The model under review builds one solid part; all positions refer to its coordinate system, in mm. Face numbers are marked on the shaded views. A direction names the side the tool comes from. Coordinates: 2 decimals unless noted, no trailing zeros. Order: outer loops, then holes, each group sorted by start corner. A loop starts at its lowest first (then second) coordinate and runs counter-clockwise, first axis right, second up. Notation, with made-up numbers: M 23.25,-21 L 46.25,-21 A21 cw 46.25,9 Z; hole C -9,78.5 d10. An arc over 180 degrees is marked long. One line per item, written item: value.
```python
from build123d import *

# Parameters (mm, degrees)
BOSS_EXTRUDE1_DEPTH        = 12.5
FILLET1_R                  = 2
F_3_5_3_5_DIAMETER_HOLE1_D = 3.5


with BuildPart() as part:
    # Sketch1 → Boss-Extrude1 (new body, symmetric)
    with BuildSketch(Plane.XY):
        Polygon((0, 0), (-18, 0), (-18, -5.5), (-35, -5.5), (-35, -3.5), (-20, -3.5), (-20, 2), (0, 2), align=None)
    extrude(amount=BOSS_EXTRUDE1_DEPTH, both=True)

    # Fillet1
    fillet1_edges = [part.edges().sort_by_distance(p)[0] for p in [
        (-18, -5.5, 0),
        (-20, 2, 0),
    ]]
    fillet(fillet1_edges, radius=FILLET1_R)

    # Ø3.5 (3.5) Diameter Hole1 (through all)
    with Locations(Plane(origin=(0, 2, 0), x_dir=(-1, 0, 0), z_dir=(0, 1, 0))):
        with Locations((5, -7.5), (5, 7.5)):
            Hole(F_3_5_3_5_DIAMETER_HOLE1_D / 2)


solid = part.part
```
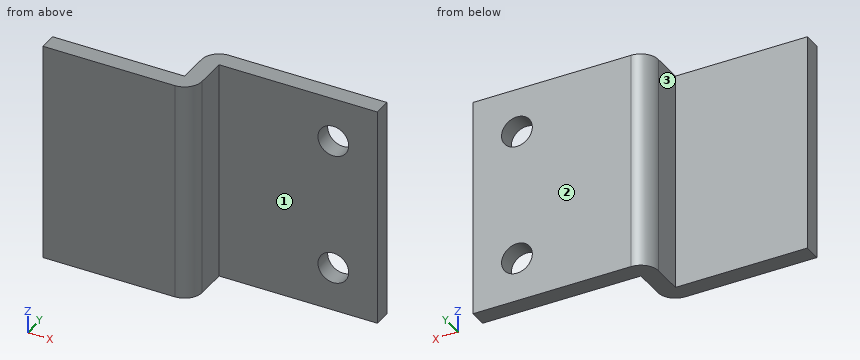
(1) Tool access review of the marked faces 1, 2 and 3: name each direction out of +Z, -Z, +X, -X, +Y, -Y from which nothing blocks a thin tool from reaching the whole face with its end or side.
Geometry results:
face 1: +Z, -Z, +X, -Y
face 2: +Z, -Z, +X, -X, +Y
face 3: +Z, -Z, -X, +Y
(2) We need section B-B, the plane z = -7.5. State the section outline as (x, y) points, plus the area to 3 significant figures.
Geometry results:
outline: M -35,-5.5 L -20,-5.5 A2 ccw -18,-3.5 L -18,0 L -6.75,0 L -6.75,2 L -18,2 A2 ccw -20,0 L -20,-3.5 L -35,-3.5 Z; M -3.25,0 L 0,0 L 0,2 L -3.25,2 Z
area: 72.3 mm2
(3) We need section C-C, the plane y = 1. State the section outline as (x, z) points, plus the area to 3 significant figures.
Geometry results:
outline: M -19.73,-12.5 L 0,-12.5 L 0,12.5 L -19.73,12.5 Z; hole C -5,-7.5 d3.5; hole C -5,7.5 d3.5
area: 474 mm2
(4) We need section A-A, the plane x = -5. State the section outline as (y, z) points.
Geometry results:
outline: M 0,-12.5 L 2,-12.5 L 2,-9.25 L 0,-9.25 Z; M 0,-5.75 L 2,-5.75 L 2,5.75 L 0,5.75 Z; M 0,9.25 L 2,9.25 L 2,12.5 L 0,12.5 Z
(5) Insertion check: pin 1 Ø8 at (x, z) = (-21, 0.5) entering from +Y; pin 2 Ø3 at (x, z) = (-5, 7.5) entering from -Y; pin 3 Ø9 at (x, z) = (-12.5, -3.5) entering from -Y; pin 4 Ø1 at (y, z) = (-1, 0.5) entering from +X. Each pin has a flat end and moves straight along its axis. Give the tip position at first contact, or say it passes through.
Geometry results:
pin 1: stops at y = 2
pin 2: passes through
pin 3: stops at y = 0
pin 4: stops at x = -18
(6) For L1, parallel to Z at x = -5, y = 0.6; L2, parallel to Y at x = -8.5, z = -8.5; L3, parallel to Y at x = -25, z = 4, list the stretches that pass through material, from the lowest coordinate up.
Geometry results:
L1: z = -12.5 to -9.25, -5.75 to 5.75, 9.25 to 12.5
L2: y = 0 to 2
L3: y = -5.5 to -3.5
(7) We need section D-D, the plane x = -16. State the section outline as (y, z) points.
Geometry results:
outline: M 0,-12.5 L 2,-12.5 L 2,12.5 L 0,12.5 Z
